Can you work these out from the drawing? Everything is in mm from the part's minimum corner. A direction names the side the tool comes from. Coordinates: 2 decimals unless noted, no trailing zeros. Loops run counter-clockwise (first coordinate to the right, second up) from the corner with the lowest first, then second, coordinate; pieces in that order, holes last. Notation, with made-up numbers: (68, 44) - (81, 44) arc R32 cw to (81, 74) - close; hole circle Ø11 at (28.5, 30). An arc over 180 degrees is marked (long way). One line per question, with ' | ' between items. Start each with the question number.
1. We'd pull the mould along Z, two halves only. Please class the marked faces 1 and 2: pulls with the +Z half, pulls with the -Z half, needs draft (parallel to the pull), parting line crosses it, or undercut.
2. I want a section at C-C, the plane x = 16.5. Write out the boundary of the cut face in (y, z).
3. I want a section at D-D, the plane z = 30.5. Write out the boundary of the cut face in (x, y).
4. I'm going to push flat-ended pins straight in: P1, Ø2.5, axis at x = 63, y = 1.5, coming from the +Z side; P2, Ø1.5, axis at x = 12.5, y = 1.5, coming from the -Z side; P3, Ø2.5, axis at x = 34, y = 3.5, coming from the -Z side; P4, Ø5, axis at x = 60, z = 30.5, coming from the +Y side. Where does each tip first touch, or does it pass through?
5. Please list where these lines run through material, in increasing order: L1, parallel to Z at x = 58, y = 4.5; L2, parallel to Z at x = 63, y = 1.3; L3, parallel to X at y = 2.85, z = 31.5. Write a range as [from, to].
6. Which directions (+Z, -Z, +X, -X, +Y, -Y) give clear straight access to the entire face, cutting with the end or side of a thin tool? Please do the marked faces 3 and 4.
7. I want a section at A-A, the plane z = 19. Write out the boundary of the cut face in (x, y).
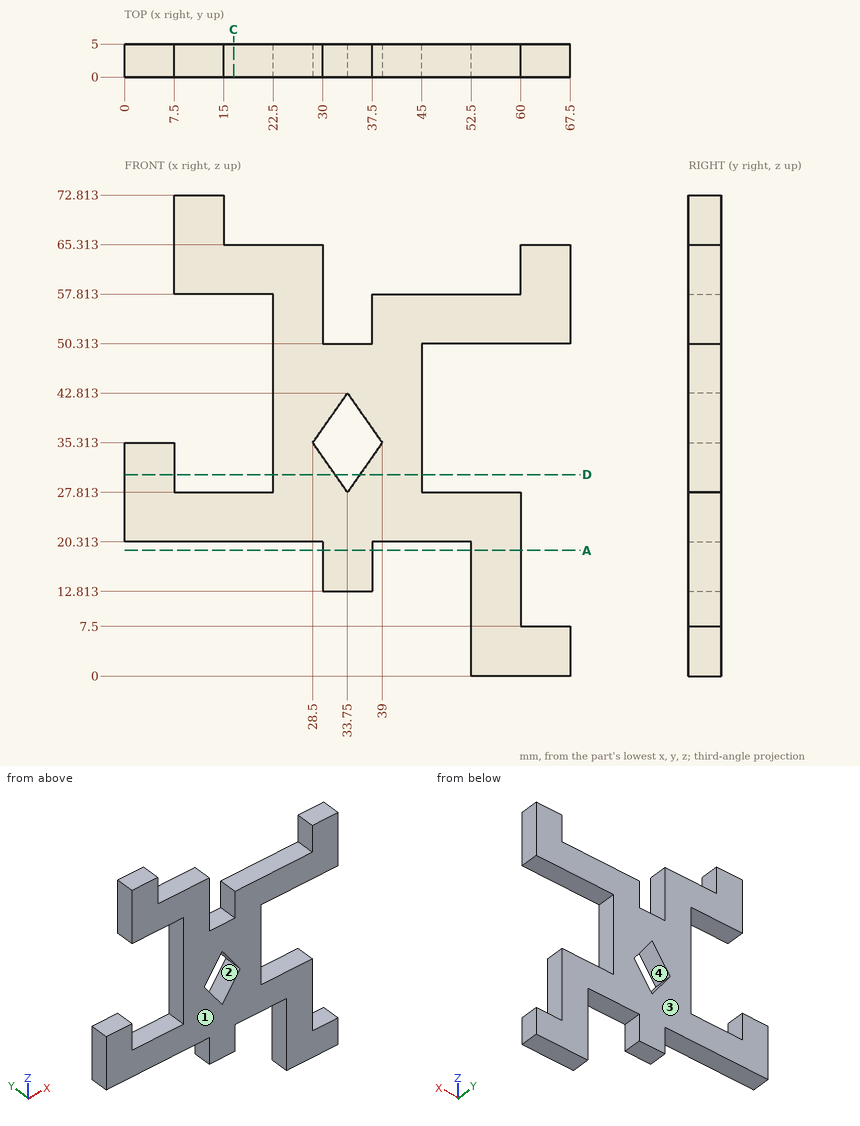
Results are:
1) face 1: needs draft | face 2: undercut
2) outline: (0, 20.31) - (5, 20.31) - (5, 27.81) - (0, 27.81) - close; (0, 57.81) - (5, 57.81) - (5, 65.31) - (0, 65.31) - close
3) outline: (0, 0) - (7.5, 0) - (7.5, 5) - (0, 5) - close; (22.5, 0) - (31.87, 0) - (31.87, 5) - (22.5, 5) - close; (35.63, 0) - (45, 0) - (45, 5) - (35.63, 5) - close
4) P1: stops at z = 65.31 | P2: stops at z = 20.31 | P3: stops at z = 12.81 | P4: passes through
5) L1: z = [0, 27.81], [50.31, 57.81] | L2: z = [0, 7.5], [50.31, 65.31] | L3: x = [0, 7.5], [22.5, 31.17], [36.33, 45]
6) face 3: +Z, -Z, +X, -X, +Y | face 4: +Y, -Y
7) outline: (30, 0) - (37.5, 0) - (37.5, 5) - (30, 5) - close; (52.5, 0) - (60, 0) - (60, 5) - (52.5, 5) - close
